from build123d import *

# Parameters (mm, degrees)
F0_R     = 37.5
F0_R_2   = 25
F1_DEPTH = 41
F3_DEPTH = 41


with BuildPart() as f1:
    # F0 (on Front) → F1 (new body)
    with BuildSketch(Plane.XZ):
        with Locations((-37.331857, -12.628307)):
            Circle(F0_R)
        with Locations((-37.331857, -12.628307)):
            Circle(F0_R_2, mode=Mode.SUBTRACT)
    extrude(amount=F1_DEPTH)

    # F2 (on face) → F3 (join)
    with BuildSketch(Plane.XZ.offset(41)):
        with BuildLine():
            Line((37.671292, -20.628307), (37.671292, -12.628307))
            Line((37.671292, -12.628307), (37.671292, -4.628307))
            Line((37.671292, -4.628307), (-0.695127, -4.628307))
            ThreePointArc((-0.695127, -4.628307), (-0.048299, -8.605085), (0.168143, -12.628307))
            ThreePointArc((0.168143, -12.628307), (-0.048299, -16.651528), (-0.695127, -20.628307))
            Line((-0.695127, -20.628307), (37.671292, -20.628307))
        make_face()
    extrude(amount=-F3_DEPTH)


solid = f1.part
Could you check a few things on this model? Use its own coordinates, in mm. A direction names the side the tool comes from. Coordinates: 2 decimals unless noted, no trailing zeros. Loops run counter-clockwise (first coordinate to the right, second up) from the corner with the lowest first, then second, coordinate; pieces in that order, holes last. Notation, with made-up numbers: (78, -29.75) -> (136, -29.75) arc R34 ccw to (136, 0.25) -> close; hole circle Ø8 at (22, 23.25). An arc over 180 degrees is marked (long way). Answer in a Markdown table with one row per item.
(1) Imagine slicing it at D-D (x = -10.5). List the corners of the cut face in (y, z) for me, plus the area to 3 significant figures.
Results found:
| item | result |
|---|---|
| outline | (-41, -38.83) -> (0, -38.83) -> (0, 13.57) -> (-41, 13.57) -> close |
| area | 2,150 mm^2 |
(2) If I drill on probe 1 along Z at (x, y) = (8, -25); probe 2 along Z at (x, y) = (-15, -24.5); probe 3 along Z at (x, y) = (-43.5, -37.5), over which ranges is the centre line in solid material (lowest first)?
Results found:
| item | result |
|---|---|
| probe 1 | z = -20.63 to -4.63 |
| probe 2 | z = -42.75 to -23.87, -1.39 to 17.5 |
| probe 3 | z = -49.62 to -36.86, 11.6 to 24.36 |
(3) Imagine slicing it at C-C (y = -36). List the corners of the cut face in (x, z) for me, plus the area to 3 significant figures.
Results found:
| item | result |
|---|---|
| outline | (-0.7, -20.63) -> (37.67, -20.63) -> (37.67, -4.63) -> (-0.7, -4.63) arc R37.5 ccw (long way) to start; hole circle Ø50 at (-37.33, -12.63) |
| area | 3,060 mm^2 |
(4) Imagine slicing it at A-A (z = -6.5). List the corners of the cut face in (x, y) for me, plus the area to 3 significant figures.
Results found:
| item | result |
|---|---|
| outline | (-74.33, -41) -> (-61.57, -41) -> (-61.57, 0) -> (-74.33, 0) -> close; (-13.09, -41) -> (37.67, -41) -> (37.67, 0) -> (-13.09, 0) -> close |
| area | 2,600 mm^2 |
(5) For faces 5 (the face through (-7, 0, -12)), 6 (the face through (19, -21, -4.628)), which set-ups out of +Z, -Z, +X, -X, +Y, -Y let a thin tool reach every point of the face, with its end or its side?
Results found:
| item | result |
|---|---|
| face 5 | +Z, -Z, +X, -X, +Y |
| face 6 | +Z, +X, +Y, -Y |
(6) Imagine slicing it at B-B (x = -47). List the corners of the cut face in (y, z) for me, plus the area to 3 significant figures.
Results found:
| item | result |
|---|---|
| outline | (-41, -48.86) -> (0, -48.86) -> (0, -35.68) -> (-41, -35.68) -> close; (-41, 10.43) -> (0, 10.43) -> (0, 23.6) -> (-41, 23.6) -> close |
| area | 1,080 mm^2 |
(7) Thinking about a two-plate mould opening in X: for faces 1 (the face through (-74.8, -20.2, -11.1)), 2 (the face through (18, -21, -20.628)), 3 (the face through (37.671, -21, -13)), 4 (the face through (-13.486, -20.213, -5.119)), which applies, released by +X, released by -X, zero draft, split by the parting line, or undercut?
Results found:
| item | result |
|---|---|
| face 1 | split by the parting line |
| face 2 | zero draft |
| face 3 | released by +X |
| face 4 | undercut |
(8) Will these pins go through, and if not, where does the flat tip stop? pin 1 Ø6 at (x, y) = (-7, -10.5) entering from -Z; pin 2 Ø1.5 at (y, z) = (-34.5, 11.5) entering from +X; pin 3 Ø12 at (y, z) = (-19, -40) entering from -X.
Results found:
| item | result |
|---|---|
| pin 1 | stops at z = -38.3 |
| pin 2 | stops at x = -8.01 |
| pin 3 | stops at x = -68.15 |
